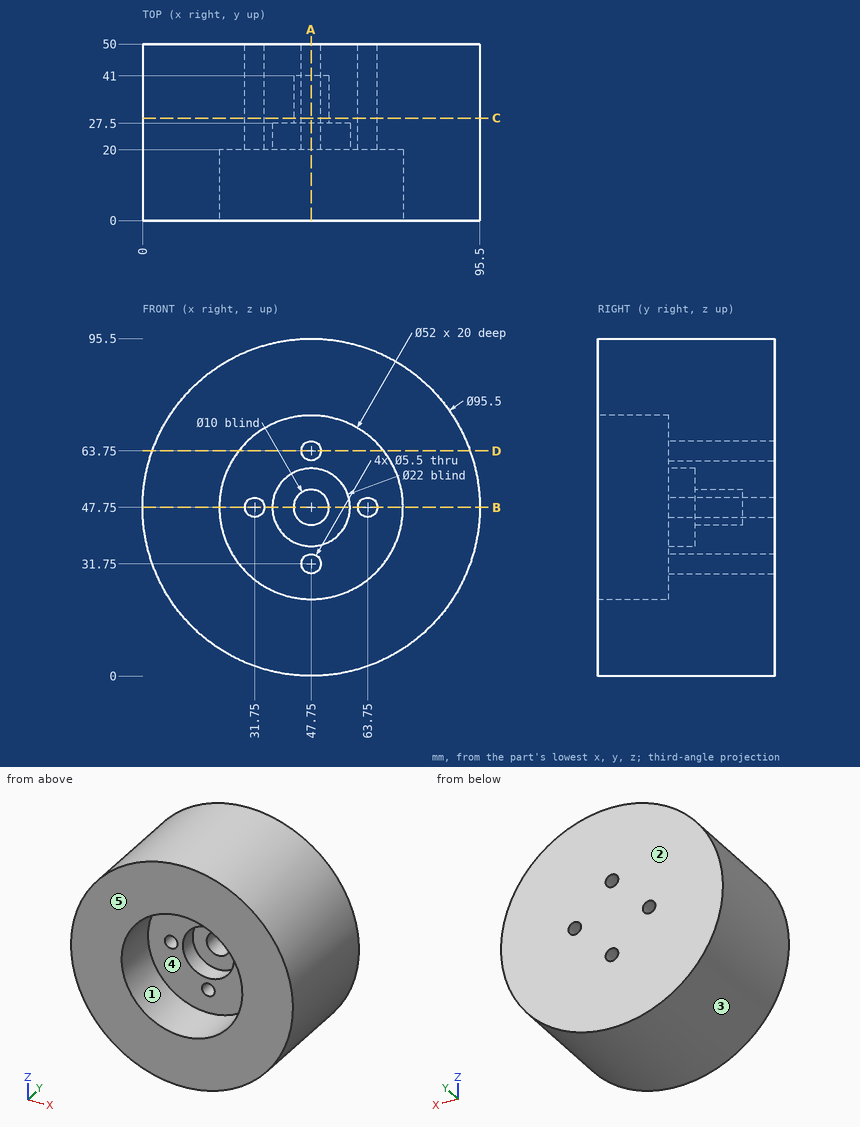
Could you check a few things on this drawing? It's one solid part, dimensions in mm from its lowest x, y, z. A direction names the side the tool comes from. Give positions to 0.01 mm unless a question says otherwise; leave off trailing zeros. Order: outer loops, then holes, each group sorted by start corner. A loop starts at its lowest first (then second) coordinate and runs counter-clockwise, first axis right, second up. Notation, with made-up numbers: M 29.5,5.5 L 81.5,5.5 A11 ccw 81.5,13.5 Z; hole C 23,-32 d4. An arc over 180 degrees is marked long. Use one line per item in the form item = value.
Item 1: For the marked faces 4 and 5, which set-ups out of +Z, -Z, +X, -X, +Y, -Y let a thin tool reach every point of the face, with its end or its side?
Values follow:
face_4 = -Y
face_5 = +Z, -Z, +X, -X, -Y
Item 2: If we section it at C-C, the plane y = 29: Write out the boundary of the cut face in (x, z), and give its area (3 significant figures).
Values follow:
outline = C 47.75,47.75 d95.5; hole C 31.75,47.75 d5.5; hole C 47.75,47.75 d10; hole C 47.75,31.75 d5.5; hole C 47.75,63.75 d5.5; hole C 63.75,47.75 d5.5
area = 6,990 mm^2
Item 3: If I drill on line 1 along X through (y, z) = (14, 47); line 2 along X through (y, z) = (37, 47); line 3 along Y through (x, z) = (44, 44), over which ranges is the centre line in solid material (lowest first)? Write a range as [from, to].
Values follow:
line_1 = [0.01, 21.76], [73.74, 95.49]
line_2 = [0.01, 29.1], [34.4, 42.81], [52.69, 61.1], [66.4, 95.49]
line_3 = [27.5, 50]
Item 4: Thinking about a two-plate mould opening in Z: for the marked faces 1, 2 and 3, which applies, pulls with the +Z half, pulls with the -Z half, needs draft (parallel to the pull), parting line crosses it, or undercut?
Values follow:
face_1 = undercut
face_2 = needs draft
face_3 = parting line crosses it
Item 5: If we section it at A-A, the plane x = 47.75: Write out the boundary of the cut face in (y, z).
Values follow:
outline = M 0,0 L 50,0 L 50,29 L 20,29 L 20,21.75 L 0,21.75 Z; M 0,73.75 L 20,73.75 L 20,66.5 L 50,66.5 L 50,95.5 L 0,95.5 Z; M 20,34.5 L 50,34.5 L 50,61 L 20,61 L 20,58.75 L 27.5,58.75 L 27.5,52.75 L 41,52.75 L 41,42.75 L 27.5,42.75 L 27.5,36.75 L 20,36.75 Z
Item 6: Will these pins go through, and if not, where does the flat tip stop? pin 1 Ø8 at (x, z) = (47.75, 47.75) entering from -Y; pin 2 Ø5 at (x, z) = (50, 46) entering from -Y; pin 3 Ø24 at (x, z) = (49, 50) entering from -Y; pin 4 Ø1.5 at (x, z) = (42.5, 79) entering from -Y.
Values follow:
pin_1 = 41
pin_2 = 27.5
pin_3 = 20
pin_4 = 0
Item 7: If we section it at B-B, the plane z = 47.75: Write out the boundary of the cut face in (x, y).
Values follow:
outline = M 0,0 L 21.75,0 L 21.75,20 L 29,20 L 29,50 L 0,50 Z; M 34.5,20 L 36.75,20 L 36.75,27.5 L 42.75,27.5 L 42.75,41 L 52.75,41 L 52.75,27.5 L 58.75,27.5 L 58.75,20 L 61,20 L 61,50 L 34.5,50 Z; M 66.5,20 L 73.75,20 L 73.75,0 L 95.5,0 L 95.5,50 L 66.5,50 Z
Item 8: If we section it at D-D, the plane z = 63.75: Write out the boundary of the cut face in (x, y), and give its area (3 significant figures).
Values follow:
outline = M 2.76,0 L 27.26,0 L 27.26,20 L 45,20 L 45,50 L 2.76,50 Z; M 50.5,20 L 68.24,20 L 68.24,0 L 92.74,0 L 92.74,50 L 50.5,50 Z
area = 3,510 mm^2
